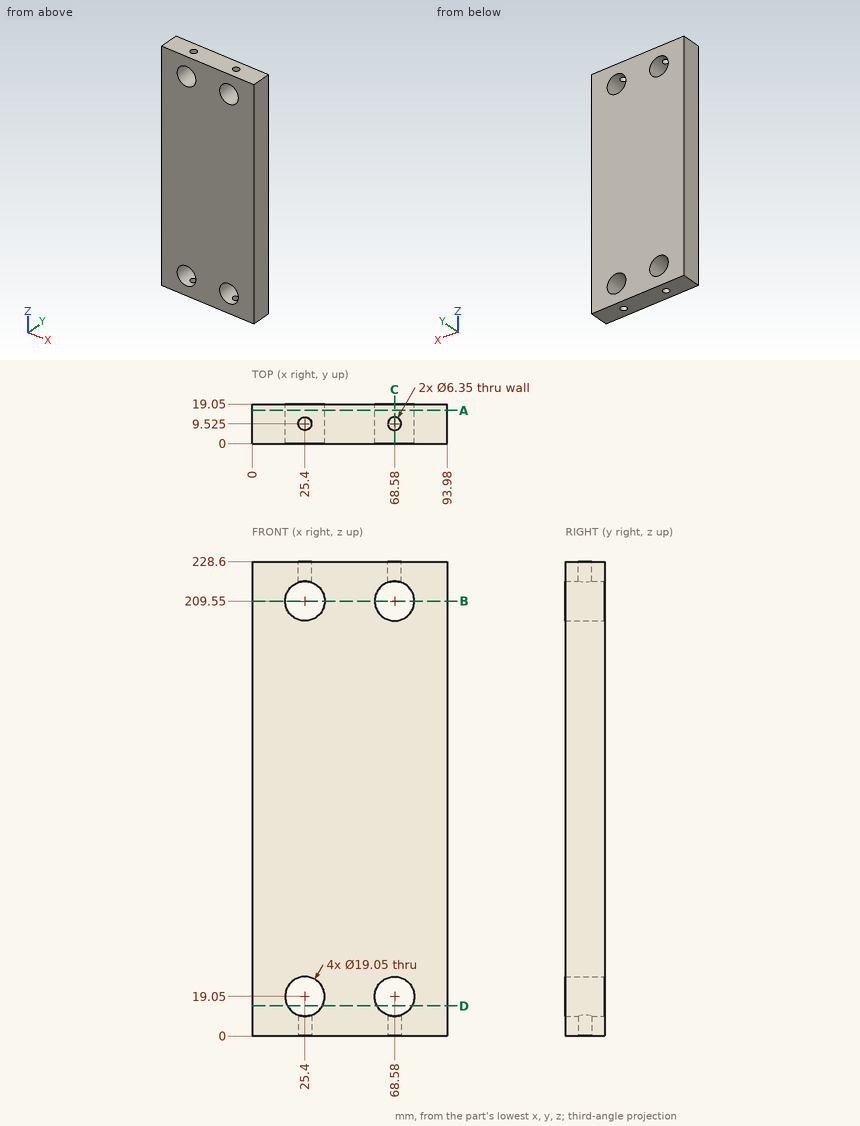
Here's the drawing with two shaded views (mm, measured from the low corner). I have some questions. Give positions to 0.01 mm unless a question says otherwise; leave off trailing zeros. Loops run counter-clockwise (first coordinate to the right, second up) from the corner with the lowest first, then second, coordinate; pieces in that order, holes last. Notation, with made-up numbers: M -23,37.25 L -19,37.25 A10 ccw -19,45.25 Z; hole C -15.5,20 d9. An arc over 180 degrees is marked long. One line per item, written item: value.
(1) Suppose I cut it at D-D on z = 14.5. List the corners of the cut face in (x, y) for me, plus the area to 3 significant figures.
Returned:
outline: M 0,0 L 17.03,0 L 17.03,19.05 L 0,19.05 Z; M 33.77,0 L 60.21,0 L 60.21,19.05 L 33.77,19.05 Z; M 76.95,0 L 93.98,0 L 93.98,19.05 L 76.95,19.05 Z
area: 1,150 mm^2
(2) I need wall thicknesses on line 1 (X direction, y = 14.5, z = 19.5); line 2 (Z direction, x = 68.58, y = 5.5) (3 decimals); line 3 (X direction, y = 11.5, z = 206). Which ranges of each line are inside material? Lowest first, please.
Returned:
line 1: 0 to 15.89, 34.91 to 59.07, 78.09 to 93.98
line 2: 0 to 9.525, 28.575 to 200.025, 219.075 to 228.6
line 3: 0 to 16.56, 34.24 to 59.74, 77.42 to 93.98
(3) Suppose I cut it at C-C on x = 68.58. List the corners of the cut face in (y, z) for me (3 decimals).
Returned:
outline: M 0,0 L 6.35,0 L 6.35,9.525 L 0,9.525 Z; M 0,28.575 L 19.05,28.575 L 19.05,200.025 L 0,200.025 Z; M 0,219.075 L 6.35,219.075 L 6.35,228.6 L 0,228.6 Z; M 12.7,0 L 19.05,0 L 19.05,9.525 L 12.7,9.525 Z; M 12.7,219.075 L 19.05,219.075 L 19.05,228.6 L 12.7,228.6 Z
(4) Suppose I cut it at A-A on y = 16. List the corners of the cut face in (x, z) for me (3 decimals), plus the area to 3 significant figures.
Returned:
outline: M 0,0 L 93.98,0 L 93.98,228.6 L 0,228.6 Z; hole C 25.4,19.05 d19.05; hole C 25.4,209.55 d19.05; hole C 68.58,19.05 d19.05; hole C 68.58,209.55 d19.05
area: 20,300 mm^2
(5) Suppose I cut it at B-B on z = 209.55. List the corners of the cut face in (x, y) for me (3 decimals), plus the area to 3 significant figures.
Returned:
outline: M 0,0 L 15.875,0 L 15.875,19.05 L 0,19.05 Z; M 34.925,0 L 59.055,0 L 59.055,19.05 L 34.925,19.05 Z; M 78.105,0 L 93.98,0 L 93.98,19.05 L 78.105,19.05 Z
area: 1,060 mm^2
(6) Will these pins go through, and if not, where does the flat tip stop? pin 1 (5.5 mm diameter, centred on x = 68.58, y = 9.525, fed in from -Z); pin 2 (17 mm diameter, centred on x = 25.4, z = 209.55, fed in from -Y); pin 3 (5 mm diameter, centred on x = 68.58, y = 9.525, fed in from +Z).
Returned:
pin 1: z = 28.17
pin 2: through
pin 3: z = 200.36
